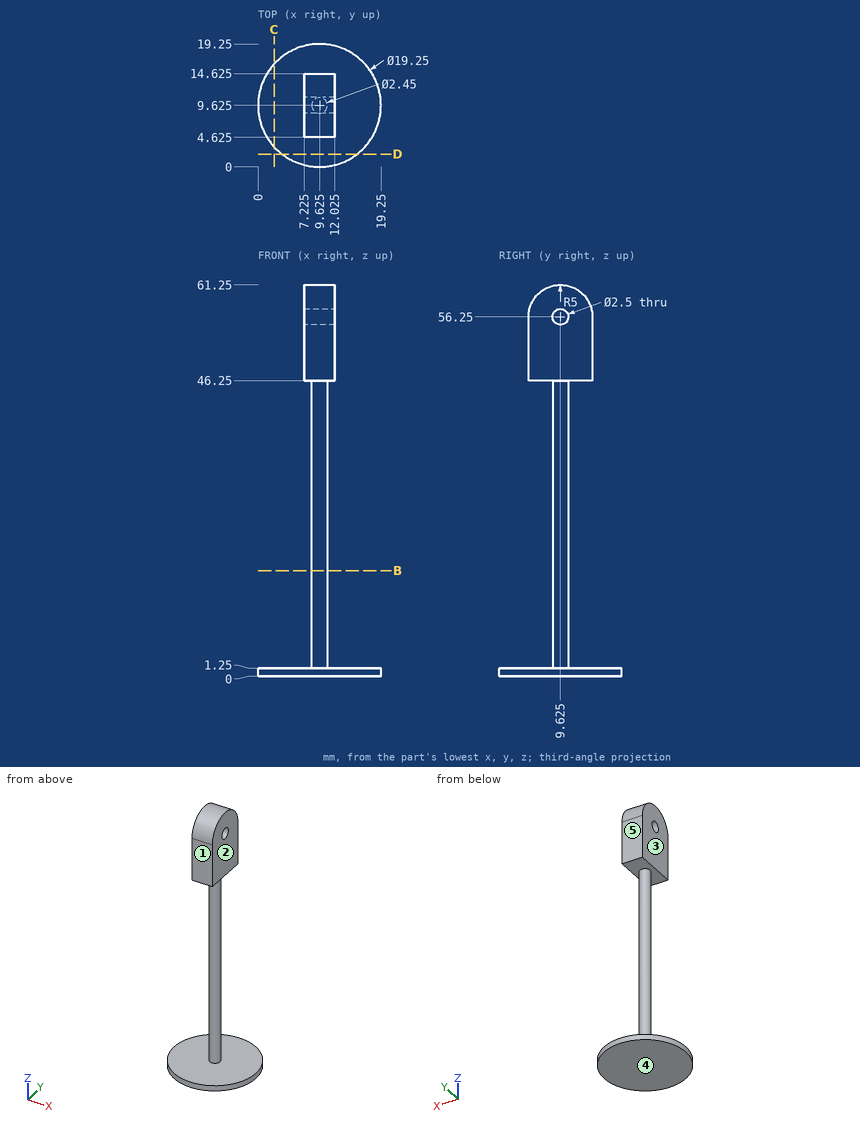
Design review of the part shown in the three views and the two pictorial views. Dimensions are in mm from the part's minimum x, y and z. A direction names the side the tool comes from. Round coordinates to 2 decimals unless told otherwise and drop trailing zeros. Write each loop counter-clockwise with the first axis right and the second up, starting at its lowest first coordinate (ties: lowest second). Pieces come first, ordered by that corner, then holes.
Item 1: For pin 1 Ø11 at (y, z) = (10.5, 54) entering from +X (3 decimals); pin 2 Ø5 at (x, z) = (11, 51) entering from -Y (3 decimals); pin 3 Ø1.4 at (x, y) = (9.5, 9) entering from -Z; pin 4 Ø5.5 at (x, z) = (8.5, 49) entering from +Y (3 decimals), all flat-tipped, find the tip position at first contact; note any pin that passes through.
Item 2: Consider section D-D on y = 2. Give the boundary of the cut face in (x, z), and give its area (3 significant figures).
Item 3: For the marked faces 1, 2, 3, 4 and 5, list the 3-axis set-ups (+Z, -Z, +X, -X, +Y, -Y) from which the entire face can be reached by the end or side of a thin tool; tool diameter is ignored.
Item 4: Consider section B-B on z = 16.5. Give the boundary of the cut face in (x, y) (3 decimals), and give its area (3 significant figures).
Item 5: Wall thickness on L1, parallel to Y at x = 8.85, z = 56.25 (3 decimals); L2, parallel to Z at x = 11, y = 9; L3, parallel to Z at x = 16.25, y = 16: over which ranges is each line inside the solid? List them lowest first.
Item 6: Consider section C-C on x = 2.5. Give the boundary of the cut face in (y, z), and give its area (3 significant figures).
Check values:
1. pin 1: stops at x = 12.025
1. pin 2: stops at y = 4.625
1. pin 3: stops at z = 0
1. pin 4: stops at y = 14.625
2. outline: (3.75, 0) - (15.5, 0) - (15.5, 1.25) - (3.75, 1.25) - close
2. area: 14.7 mm2
3. face 1: +Z, +X, -X, -Y
3. face 2: +Z, +X, +Y, -Y
3. face 3: +Z, -X, +Y, -Y
3. face 4: -Z, +X, -X, +Y, -Y
3. face 5: +Z, +X, -X, +Y
4. outline: circle Ø2.45 at (9.625, 9.625)
4. area: 4.71 mm2
5. L1: y = 4.625 to 8.375, 10.875 to 14.625
5. L2: z = 0 to 1.25, 46.25 to 55.17, 57.33 to 61.21
5. L3: z = 0 to 1.25
6. outline: (3.15, 0) - (16.1, 0) - (16.1, 1.25) - (3.15, 1.25) - close
6. area: 16.2 mm2
